Verification items for the finished model (mm, model axes). Face numbers are marked on the shaded views. A direction names the side the tool comes from. Coordinates: 2 decimals unless noted, no trailing zeros. Order: outer loops, then holes, each group sorted by start corner. A loop starts at its lowest first (then second) coordinate and runs counter-clockwise, first axis right, second up. Notation, with made-up numbers: M 69,35.5 L 96,35.5 A14 ccw 96,62.5 Z; hole C -40,16 d2. An arc over 180 degrees is marked long. Return JSON: item names as keys, results as strings.
```python
from build123d import *

# Parameters (mm, degrees)
F0_W = 54.543138
F0_H = 44.022134


with BuildPart() as f1:
    # F0 (on Top) → F1 (revolve)
    with BuildSketch(Plane.XY):
        Polygon((-1250, 150), (-1250, 0), (1250, 0), (1250, 150), (964.447558, 150), (909.90442, 150), (833.874702, 150), (76.882489, 150), (-86.746827, 150), (-374.337733, 150), (-637.13634, 150), (-1123.065829, 150), align=None)
        Polygon((-1060.258627, 197.327778), (-1123.065829, 150), (-637.13634, 150), (-668.539941, 177.4939), (-802.41847, 177.4939), (-858.614385, 230.384186), (-946.213901, 230.384186), (-946.213901, 197.327778), align=None)
        with Locations((937.175989, 172.011067)):
            Rectangle(F0_W, F0_H)
        Polygon((-374.337733, 189.063668), (-374.337733, 150), (-86.746827, 150), (-86.746827, 189.063668), (-119.80325, 189.063668), (-119.80325, 235.342652), (-336.322844, 235.342652), (-336.322844, 189.063668), align=None)
        Polygon((76.882489, 150), (833.874702, 150), (693.384826, 182.452381), (207.455367, 182.452381), align=None)
    revolve(axis=Axis((0, 0, 0), (1, 0, 0)))


solid = f1.part
```
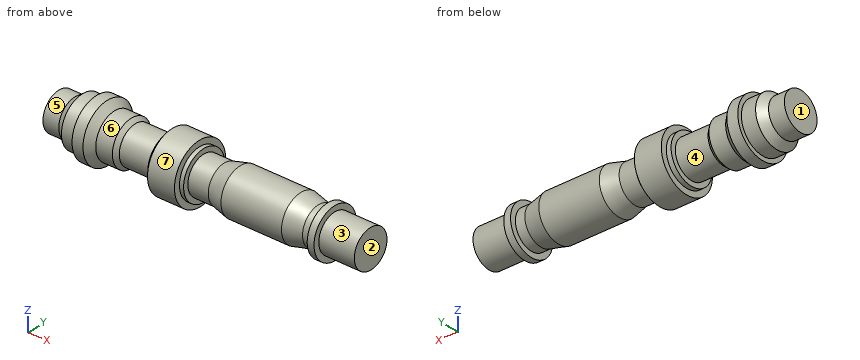
Q1. Go/stop test with flat-tipped pins: pin 1 (12 mm diameter, centred on y = 130.5, z = 150, fed in from -X); pin 2 (10 mm diameter, centred on x = -861.5, z = 177.5, fed in from -Y); pin 3 (2 mm diameter, centred on x = -843, y = 64.5, fed in from +Z). Record where each tip stops, or that it passes through.
Values:
{"pin 1": "x = -1066.24", "pin 2": "y = -152.71", "pin 3": "z = 206.85"}
Q2. Material ranges on line 1 along X through (y, z) = (-187, -24); line 2 along X through (y, z) = (145.5, -182); line 3 along X through (y, z) = (64.5, 193), recorded low to high.
Values:
{"line 1": "-1071.93 to -814.15, -374.34 to -86.75, 909.9 to 964.45", "line 2": "-336.32 to -119.8", "line 3": "-946.21 to -830.04, -336.32 to -119.8"}
Q3. Cross-section at A-A, the plane x = -775. Record the boundary of the cut face in (y, z).
Values:
{"outline": "C 0,0 d354.99"}
Q4. Draft check along X on the marked faces 1, 2, 3 and 4. Enter one of: pulls with the +X half, pulls with the -X half, needs draft (parallel to the pull), parting line crosses it, or undercut.
Values:
{"face 1": "pulls with the -X half", "face 2": "pulls with the +X half", "face 3": "needs draft", "face 4": "undercut"}
Q5. Cross-section at B-B, the plane x = 754. Record the boundary of the cut face in (y, z).
Values:
{"outline": "C 0,0 d336.9"}
Q6. Tool access check on the marked faces 5, 6 and 7. Record the directions out of +Z, -Z, +X, -X, +Y, -Y that give a thin tool (end or side, any length) a straight path to the whole face; none if there is none.
Values:
{"face 5": "-X", "face 6": "none", "face 7": "+X, -X"}
